For this review, use the dimensioned drawing (mm, ordinates from the lowest corner) and the shaded views. A direction names the side the tool comes from. Give positions to 0.01 mm unless a question says otherwise; leave off trailing zeros. Order: outer loops, then holes, each group sorted by start corner. A loop starts at its lowest first (then second) coordinate and runs counter-clockwise, first axis right, second up. Notation, with made-up numbers: (56, 35.25) - (98, 35.25) arc R31 cw to (98, 74.25) - close; hole circle Ø3 at (54, 2.25). An arc over 180 degrees is marked (long way). One line per item, written item: value.
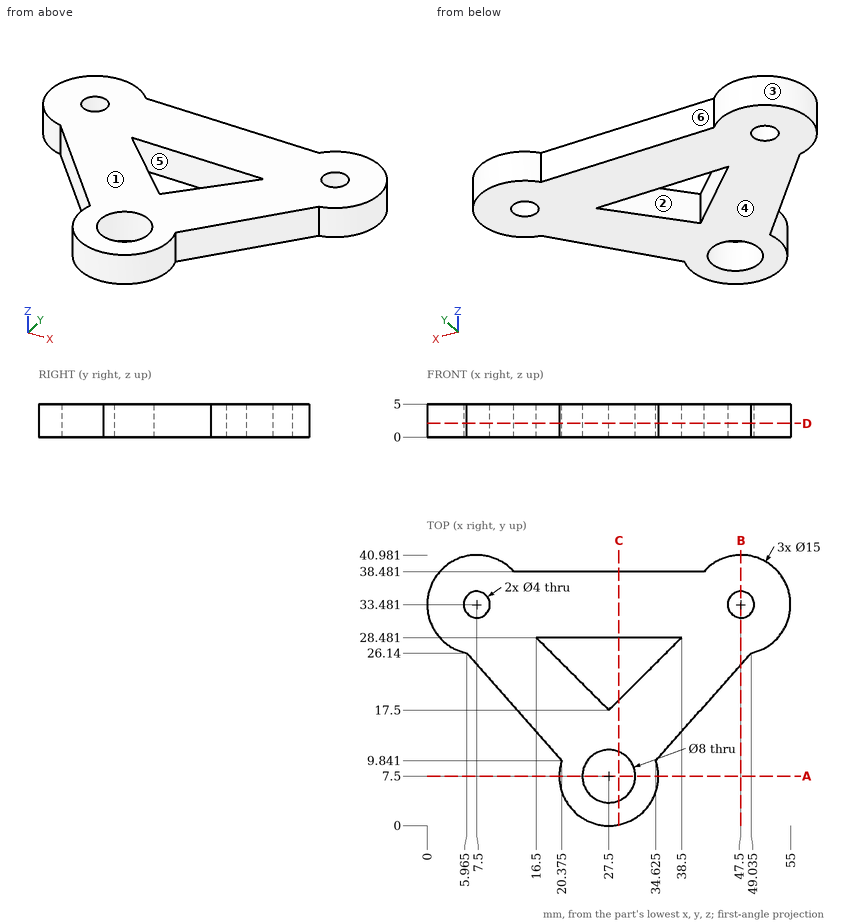
(1) Take a section at D-D (z = 2.05). Write out the cut boundary in (x, y) (1 decimal).
Answers below:
outline: (6, 26.1) - (20.4, 9.8) arc R7.5 ccw (long way) to (34.6, 9.8) - (49, 26.1) arc R7.5 ccw (long way) to (41.9, 38.5) - (13.1, 38.5) arc R7.5 ccw (long way) to start; hole circle Ø4 at (7.5, 33.5); hole (16.5, 28.5) - (27.5, 17.5) - (38.5, 28.5) - close; hole circle Ø8 at (27.5, 7.5); hole circle Ø4 at (47.5, 33.5)
(2) Take a section at A-A (y = 7.5). Write out the cut boundary in (x, z), then the cut area to 3 significant figures.
Answers below:
outline: (20, 0) - (23.5, 0) - (23.5, 5) - (20, 5) - close; (31.5, 0) - (35, 0) - (35, 5) - (31.5, 5) - close
area: 35.0 mm^2
(3) Draft analysis for pull direction Y (two halves, no side actions). For the marked faces 3, 4, 5 and 6, state which applies: pulls with the +Y half, pulls with the -Y half, needs draft (parallel to the pull), parting line crosses it, or undercut.
Answers below:
face 3: parting line crosses it
face 4: needs draft
face 5: undercut
face 6: pulls with the +Y half
(4) Take a section at C-C (x = 29). Write out the cut boundary in (y, z), then the cut area to 3 significant figures.
Answers below:
outline: (0.15, 0) - (3.79, 0) - (3.79, 5) - (0.15, 5) - close; (11.21, 0) - (19, 0) - (19, 5) - (11.21, 5) - close; (28.48, 0) - (38.48, 0) - (38.48, 5) - (28.48, 5) - close
area: 107 mm^2
(5) Take a section at B-B (x = 47.5). Write out the cut boundary in (y, z).
Answers below:
outline: (24.4, 0) - (31.48, 0) - (31.48, 5) - (24.4, 5) - close; (35.48, 0) - (40.98, 0) - (40.98, 5) - (35.48, 5) - close
(6) For P1, Ø1, axis at y = 27, z = 2, coming from the -X side (1 decimal); P2, Ø1.5, axis at y = 23.5, z = 3.5, coming from the -X side (1 decimal); P3, Ø6.5, axis at x = 27.5, y = 7.5, coming from the -Z side; P4, Ø2.5, axis at x = 21, z = 2.5, coming from the +Y side, all flat-tipped, find the tip position at first contact; note any pin that passes through.
Answers below:
P1: stops at x = 3
P2: stops at x = 7.6
P3: passes through
P4: stops at y = 38.48
(7) Machinability: for the marked faces 1 and 2, which of the approach directions +Z, -Z, +X, -X, +Y, -Y give a long, thin tool a straight path to every point of the face, cutting with its end or side? Answer none if there is none.
Answers below:
face 1: +Z, +X, -X, +Y, -Y
face 2: +Z, -Z
(8) Wall thickness on line 1 (X direction, y = 23, z = 2.7); line 2 (Y direction, x = 19, z = 4.75) (1 decimal); line 3 (X direction, y = 7, z = 0.4): over which ranges is each line inside the solid? List them lowest first. Write a range as from..to.
Answers below:
line 1: x = 8.74..21.99, 33.01..46.26
line 2: y = 11.4..26, 28.5..38.5
line 3: x = 20.02..23.53, 31.47..34.98
